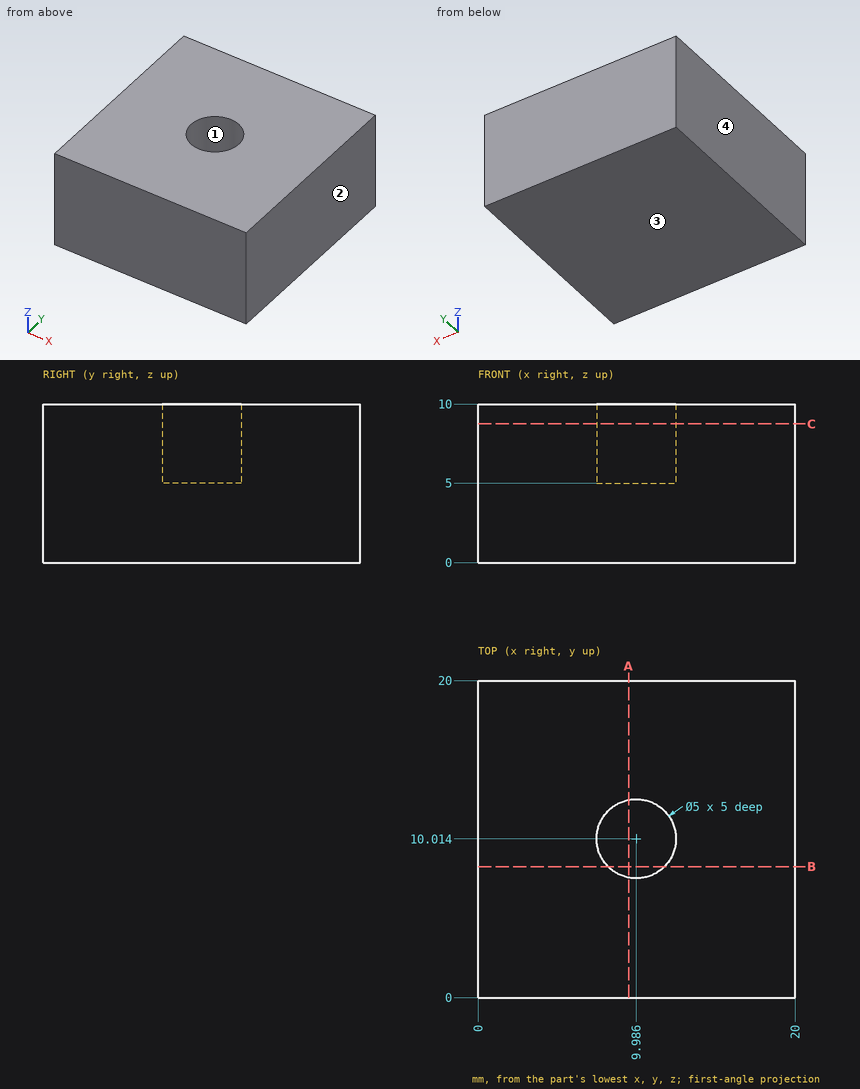
Geometry check sheet. Reference: drawing and pictorial views, mm from the part's lowest x, y, z. Round coordinates to 2 decimals unless told otherwise and drop trailing zeros. Loops run counter-clockwise (first coordinate to the right, second up) from the corner with the lowest first, then second, coordinate; pieces in that order, holes last. Notation, with made-up numbers: (56, 27) -> (70, 27) arc R17 ccw to (70, 54) -> close; hole circle Ø9 at (68.25, 41). An arc over 180 degrees is marked (long way). Answer as a JSON object with one key per item and string values.
Q1. Section check A-A (x = 9.5). Record the boundary of the cut face in (y, z).
Data:
{"outline": "(0, 0) -> (20, 0) -> (20, 10) -> (12.47, 10) -> (12.47, 5) -> (7.56, 5) -> (7.56, 10) -> (0, 10) -> close"}
Q2. Section check C-C (z = 8.75). Record the boundary of the cut face in (x, y) (1 decimal), then the cut area to 3 significant figures.
Data:
{"outline": "(0, 0) -> (20, 0) -> (20, 20) -> (0, 20) -> close; hole circle Ø5 at (10, 10)", "area": "380 mm2"}
Q3. Section check B-B (y = 8.25). Record the boundary of the cut face in (x, z) (1 decimal), then the cut area to 3 significant figures.
Data:
{"outline": "(0, 0) -> (20, 0) -> (20, 10) -> (11.8, 10) -> (11.8, 5) -> (8.2, 5) -> (8.2, 10) -> (0, 10) -> close", "area": "182 mm2"}
Q4. Draft check along X on the marked faces 1, 2, 3 and 4. Enter one of: pulls with the +X half, pulls with the -X half, needs draft (parallel to the pull), parting line crosses it, or undercut.
Data:
{"face 1": "undercut", "face 2": "pulls with the +X half", "face 3": "needs draft", "face 4": "pulls with the -X half"}
Q5. Go/stop test with a flat-tipped pin: P1, Ø2.5, axis at x = 10, y = 9, coming from the +Z side. Record where the tip stops, or that it passes through.
Data:
{"P1": "stops at z = 5"}
Q6. Scan line: line 1 (Z direction, x = 10.75, y = 8). Record every from-to range of solid material in increasing order. Write a range as from..to.
Data:
{"line 1": "z = 0..5"}
